Input: part model. Units: mm. Frame: model coordinates. Give positions to 0.01 mm unless a question says otherwise; leave off trailing zeros. Write each loop counter-clockwise with the first axis right and the second up, starting at its lowest first coordinate (ties: lowest second). Pieces come first, ordered by that corner, then holes. Notation, with made-up numbers: M 81.25,29 L 123.25,29 A18 cw 123.25,56 Z; hole C -24,54.25 d10. An arc over 180 degrees is marked long. Use CSV: the item, a comma, the result in double quotes. Start each with the question number.
from build123d import *

# Parameters (mm, degrees)
BASPROSKE_W        = 2
BASPROSKE_H        = 15
TOOTHCUT_DEPTH     = 22.307275753
TEETHCUTS_COUNT    = 28
TEETHCUTS_ANGLE    = 347.142857143
BORSKE_R           = 1.5
BORE_DEPTH         = 50.0000508
CUT_EXTRUDE1_DEPTH = 10


with BuildPart() as part:
    # BasProSke → Base-Revolve (revolve)
    with BuildSketch(Plane(origin=(0, 0, 0), x_dir=(1, 0, 0), z_dir=(0, 1, 0)), mode=Mode.PRIVATE) as base_revolve_sk:
        with Locations((1, 7.5)):
            Rectangle(BASPROSKE_W, BASPROSKE_H)
    revolve(base_revolve_sk.sketch.rotate(Axis((-10, 0, 0), (1, 0, 0)), 180), axis=Axis((-10, 0, 0), (1, 0, 0)))

    # TooCutSke → ToothCut (cut, through all)
    with BuildSketch(Plane(origin=(0, 0, 0), x_dir=(0, 0, -1), z_dir=(1, 0, 0))):
        with BuildLine():
            ThreePointArc((0.471336039, 12.740284272), (0, 12.749), (-0.471336039, 12.740284272))
            ThreePointArc((-0.471336039, 12.740284272), (-0.81983923, 13.900763331), (-1.409805137, 14.959114099))
            ThreePointArc((-1.409805137, 14.959114099), (0, 15.0254), (1.409805137, 14.959114099))
            ThreePointArc((1.409805137, 14.959114099), (0.81983923, 13.900763331), (0.471336039, 12.740284272))
        make_face()
    toothcut = extrude(amount=TOOTHCUT_DEPTH, mode=Mode.SUBTRACT)

    # TeethCuts: ToothCut ×28 about axis
    teethcuts_axis = Axis((-10, 0, 0), (1, 0, 0))
    for i in range(1, TEETHCUTS_COUNT):
        add(toothcut.rotate(teethcuts_axis, i * TEETHCUTS_ANGLE / (TEETHCUTS_COUNT - 1)), mode=Mode.SUBTRACT)

    # BorSke → Bore (cut, symmetric)
    with BuildSketch(Plane(origin=(0, 0, 0), x_dir=(0, 0, -1), z_dir=(1, 0, 0))):
        with Locations(Location((0, 0, 0), (0, 0, 180))):
            Circle(BORSKE_R)
    extrude(amount=BORE_DEPTH, both=True, mode=Mode.SUBTRACT)

    # Sketch1 → Cut-Extrude1 (cut)
    with BuildSketch(Plane(origin=(2, 0, 0), x_dir=(0, 0, -1), z_dir=(1, 0, 0))):
        with BuildLine():
            Line((0, 1.95), (1.564448785, 1.95))
            ThreePointArc((1.564448785, 1.95), (0, -2.5), (-1.564448785, 1.95))
            Line((-1.564448785, 1.95), (0, 1.95))
        make_face()
    extrude(amount=-CUT_EXTRUDE1_DEPTH, mode=Mode.SUBTRACT)


solid = part.part
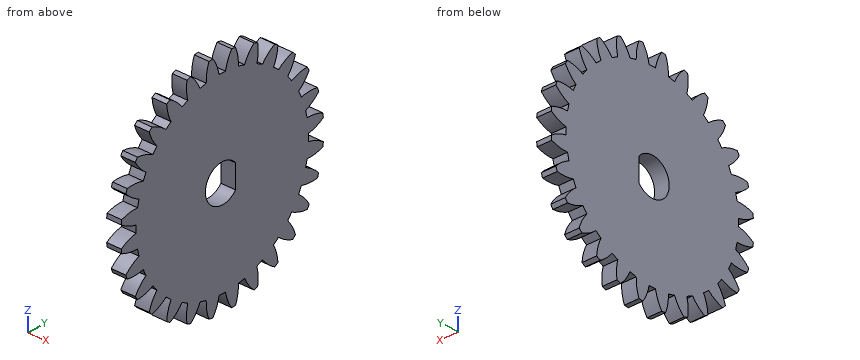
Q1. Section C-C, the plane y = -4. Return the cut outline in (x, z).
Q2. First-contact query: pin 1 Ø1 at (x, z) = (1, -8.5) entering from -Y; pin 2 Ø1 at (x, z) = (1, 0.5) entering from -Y. Flat tips, straight axial feed; report the tip coordinate or a pass-through.
Q3. Section A-A, the plane z = 0. Return the cut outline in (x, y), and give its area (3 significant figures).
Q4. Material intervals for L1, parallel to Y at x = 0.35, z = -9.75; L2, parallel to Y at x = 0.9, z = 0; L3, parallel to Z at x = 1.95, y = -12, sorted ascending. Write a range as [from, to].
Q5. Section B-B, the plane y = 0. Return the cut outline in (x, z), and give its area (3 significant figures).
Check result:
1,outline,"M 0,-13.51 L 2,-13.51 L 2,13.51 L 0,13.51 Z"
2,pin 1,"stops at y = -12.69"
2,pin 2,"stops at y = -14.29"
3,outline,"M 0,-12.75 L 2,-12.75 L 2,-2.5 L 0,-2.5 Z; M 0,1.95 L 2,1.95 L 2,12.75 L 0,12.75 Z"
3,area,"42.1 mm²"
4,L1,"y = [-10.57, -8.41], [-8.21, 8.21], [8.41, 10.57]"
4,L2,"y = [-12.75, -2.5], [1.95, 12.75]"
4,L3,"z = [-8.16, -6.59], [-5.18, 5.18], [6.59, 8.16]"
5,outline,"M 0,-12.75 L 2,-12.75 L 2,-2.5 L 0,-2.5 Z; M 0,2.5 L 2,2.5 L 2,12.75 L 0,12.75 Z"
5,area,"41.0 mm²"
